Verification items for the finished model (mm, model axes). Face numbers are marked on the shaded views. A direction names the side the tool comes from. Give positions to 0.01 mm unless a question says otherwise; leave off trailing zeros. Order: outer loops, then holes, each group sorted by start corner. A loop starts at its lowest first (then second) coordinate and runs counter-clockwise, first axis right, second up.
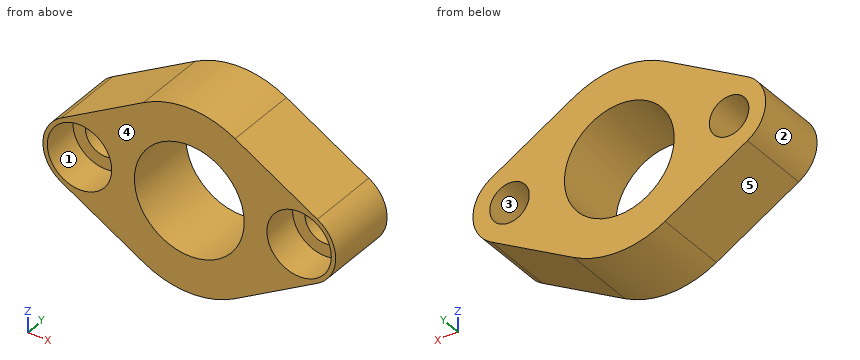
from build123d import *

# Parameters (mm, degrees)
F0_R     = 3.429
F0_R_2   = 9.525
F1_DEPTH = 12.7
F2_R     = 5.588
F2_R_2   = 3.429
F3_DEPTH = 6.35


with BuildPart() as f1:
    # F0 (on Front) → F1 (new body)
    with BuildSketch(Plane.XZ):
        with BuildLine():
            Line((-7.9375, 13.748153), (-22.225, 5.499261))
            ThreePointArc((-22.225, 5.499261), (-25.4, 0), (-22.225, -5.499261))
            Line((-22.225, -5.499261), (-7.9375, -13.748153))
            ThreePointArc((-7.9375, -13.748153), (0, -15.875), (7.9375, -13.748153))
            Line((7.9375, -13.748153), (22.225, -5.499261))
            ThreePointArc((22.225, -5.499261), (25.4, 0), (22.225, 5.499261))
            Line((22.225, 5.499261), (7.9375, 13.748153))
            ThreePointArc((7.9375, 13.748153), (0, 15.875), (-7.9375, 13.748153))
        make_face()
        with Locations((-19.05, 0)):
            Circle(F0_R, mode=Mode.SUBTRACT)
        Circle(F0_R_2, mode=Mode.SUBTRACT)
        with Locations((19.05, 0)):
            Circle(F0_R, mode=Mode.SUBTRACT)
    extrude(amount=F1_DEPTH)

    # F2 (on face) → F3 (cut)
    with BuildSketch(Plane.XZ.offset(12.7)):
        with Locations((-19.05, 0)):
            Circle(F2_R)
        with Locations((-19.05, 0)):
            Circle(F2_R_2, mode=Mode.SUBTRACT)
        with Locations((19.05, 0)):
            Circle(F2_R)
        with Locations((19.05, 0)):
            Circle(F2_R_2, mode=Mode.SUBTRACT)
    extrude(amount=-F3_DEPTH, mode=Mode.SUBTRACT)


solid = f1.part
(1) Section check A-A, the plane z = 0. Enter the section's corners in (x, y) (3 decimals), then the cut area to 3 significant figures.
Solved:
outline: (-25.4, -12.7) - (-24.638, -12.7) - (-24.638, -6.35) - (-22.479, -6.35) - (-22.479, 0) - (-25.4, 0) - close; (-15.621, -6.35) - (-13.462, -6.35) - (-13.462, -12.7) - (-9.525, -12.7) - (-9.525, 0) - (-15.621, 0) - close; (9.525, -12.7) - (13.462, -12.7) - (13.462, -6.35) - (15.621, -6.35) - (15.621, 0) - (9.525, 0) - close; (22.479, -6.35) - (24.638, -6.35) - (24.638, -12.7) - (25.4, -12.7) - (25.4, 0) - (22.479, 0) - close
area: 174 mm2
(2) Section check B-B, the plane x = 0. Enter the section's corners in (y, z) (3 decimals).
Solved:
outline: (-12.7, -15.875) - (0, -15.875) - (0, -9.525) - (-12.7, -9.525) - close; (-12.7, 9.525) - (0, 9.525) - (0, 15.875) - (-12.7, 15.875) - close
(3) Section check C-C, the plane y = -8.25. Give the number of separate pieces and of enclosed holes in the cut face, then the cut area to 3 significant figures.
Solved:
separate pieces: 1
enclosed holes: 3
area: 600 mm2
(4) Section check D-D, the plane z = 6.5. Enter the section's corners in (x, y).
Solved:
outline: (-20.49, -12.7) - (-6.96, -12.7) - (-6.96, 0) - (-20.49, 0) - close; (6.96, -12.7) - (20.49, -12.7) - (20.49, 0) - (6.96, 0) - close
(5) Go/stop test with flat-tipped pins: pin 1 (1.5 mm diameter, centred on x = 18.5, y = -3.5, fed in from +Z); pin 2 (9 mm diameter, centred on x = -17, z = -1.5, fed in from -Y); pin 3 (1 mm diameter, centred on x = 9.5, y = -11, fed in from +Z); pin 4 (6 mm diameter, centred on x = -19.05, z = 0, fed in from -Y). Record where each tip stops, or that it passes through.
Solved:
pin 1: stops at z = 8.08
pin 2: stops at y = -12.7
pin 3: stops at z = 13.13
pin 4: passes through
(6) Set-up check for the marked faces 1 and 2: record each of +Z, -Z, +X, -X, +Y, -Y from which the full face is reachable in a straight line by a thin tool's end or side.
Solved:
face 1: -Y
face 2: -X, +Y, -Y
(7) Scan lines: line 1 (Z direction, x = 0, y = -3.5) (3 decimals); line 2 (X direction, y = -10.25, z = 4.5); line 3 (Z direction, x = 19.05, y = -3.5). Record each from-to range of solid material in increasing order.
Solved:
line 1: z = -15.875 to -9.525, 9.525 to 15.875
line 2: x = -23.53 to -22.36, -15.74 to -8.39, 8.39 to 15.74, 22.36 to 23.53
line 3: z = -7.33 to -3.43, 3.43 to 7.33
(8) Release check for a two-part mould opening along Z. For the marked faces 3, 4 and 5 record: pulls with the +Z half, pulls with the -Z half, needs draft (parallel to the pull), parting line crosses it, or undercut.
Solved:
face 3: undercut
face 4: needs draft
face 5: pulls with the -Z half
